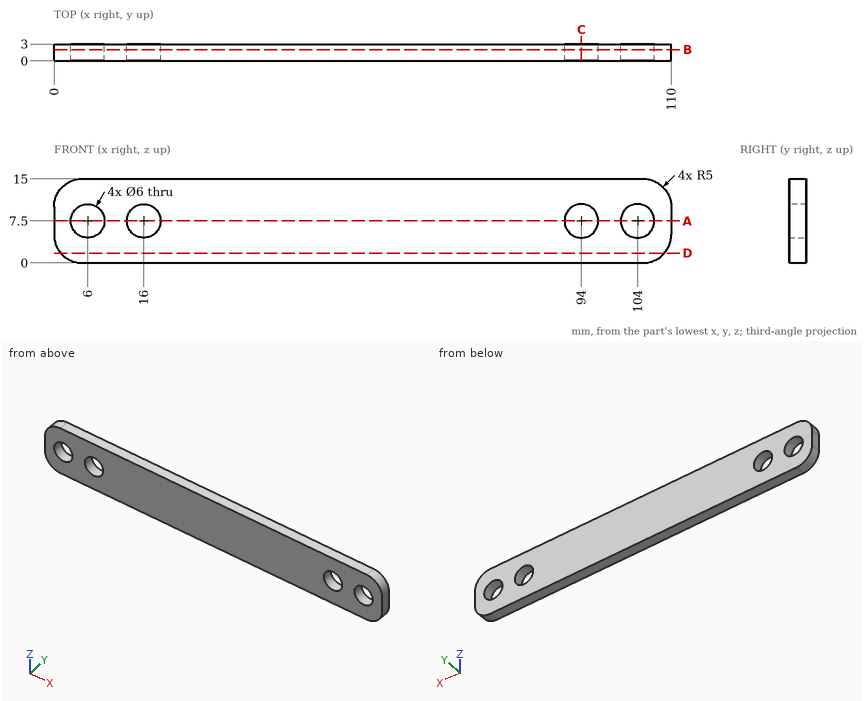
Input: dimensioned drawing with shaded views. Units: mm. Origin: part minimum x, y, z. Coordinates: 2 decimals unless noted, no trailing zeros. Order: outer loops, then holes, each group sorted by start corner. A loop starts at its lowest first (then second) coordinate and runs counter-clockwise, first axis right, second up.
1. Cut plane C-C, the plane x = 94. Return loops of the section in (y, z).
Checked values:
outline: (0, 0) - (3, 0) - (3, 4.5) - (0, 4.5) - close; (0, 10.5) - (3, 10.5) - (3, 15) - (0, 15) - close
2. Ray query, line 1 along X through (y, z) = (2.8, 7.25); line 2 along Z through (x, y) = (104, 1.8); line 3 along X through (y, z) = (1.85, 6). Return the intervals inside material, ascending.
Checked values:
line 1: x = 0 to 3.01, 8.99 to 13.01, 18.99 to 91.01, 96.99 to 101.01, 106.99 to 110
line 2: z = 0 to 4.5, 10.5 to 15
line 3: x = 0 to 3.4, 8.6 to 13.4, 18.6 to 91.4, 96.6 to 101.4, 106.6 to 110
3. Cut plane D-D, the plane z = 1.75. Return loops of the section in (x, y), plus the area to 3 significant figures.
Checked values:
outline: (1.2, 0) - (108.8, 0) - (108.8, 3) - (1.2, 3) - close
area: 323 mm2
4. Cut plane B-B, the plane y = 2. Return loops of the section in (x, z).
Checked values:
outline: (0, 5) arc R5 ccw to (5, 0) - (105, 0) arc R5 ccw to (110, 5) - (110, 10) arc R5 ccw to (105, 15) - (5, 15) arc R5 ccw to (0, 10) - close; hole circle Ø6 at (6, 7.5); hole circle Ø6 at (16, 7.5); hole circle Ø6 at (94, 7.5); hole circle Ø6 at (104, 7.5)
5. Cut plane A-A, the plane z = 7.5. Return loops of the section in (x, y).
Checked values:
outline: (0, 0) - (3, 0) - (3, 3) - (0, 3) - close; (9, 0) - (13, 0) - (13, 3) - (9, 3) - close; (19, 0) - (91, 0) - (91, 3) - (19, 3) - close; (97, 0) - (101, 0) - (101, 3) - (97, 3) - close; (107, 0) - (110, 0) - (110, 3) - (107, 3) - close
